Build history of the part. All positions in model axes, mm. A direction names the side the tool comes from. Give positions to 0.01 mm unless a question says otherwise; leave off trailing zeros. Order: outer loops, then holes, each group sorted by start corner. A loop starts at its lowest first (then second) coordinate and runs counter-clockwise, first axis right, second up. Notation, with made-up numbers: M 2.5,8.25 L 52.5,8.25 A6 ccw 52.5,13.25 Z; hole C 1.5,76 d8. An arc over 180 degrees is marked long. One line per item, written item: value. Start each with the question number.
from build123d import *

# Parameters (mm, degrees)
SKETCH1_W           = 92.3
SKETCH1_H           = 30.5
SKETCH1_W_2         = 84.3
SKETCH1_H_2         = 26.5
BOSS_EXTRUDE1_DEPTH = 3
SKETCH2_W           = 3
SKETCH2_H           = 3
BOSS_EXTRUDE2_DEPTH = 5


with BuildPart() as part:
    # Sketch1 → Boss-Extrude1 (new body)
    # profile 1 of 2: a face of its own
    with BuildSketch(Plane.XY):
        with Locations((0, 0.6)):
            Rectangle(SKETCH1_W, SKETCH1_H)
        with Locations((0, 0.6)):
            Rectangle(SKETCH1_W_2, SKETCH1_H_2, mode=Mode.SUBTRACT)
    # profile 2 of 2: a face of its own
    with BuildSketch(Plane.XY):
        with Locations((0, 0.6)):
            Rectangle(SKETCH1_W_2, SKETCH1_H_2)
    extrude(amount=BOSS_EXTRUDE1_DEPTH)

    # Sketch2 → Boss-Extrude2 (add)
    with BuildSketch(Plane.XY.offset(3)):
        with Locations((-40.65, 12.35)):
            Rectangle(SKETCH2_W, SKETCH2_H)
        with Locations((40.65, 12.35)):
            Rectangle(SKETCH2_W, SKETCH2_H)
        with Locations((40.65, -11.15)):
            Rectangle(SKETCH2_W, SKETCH2_H)
        with Locations((-40.65, -11.15)):
            Rectangle(SKETCH2_W, SKETCH2_H)
    extrude(amount=BOSS_EXTRUDE2_DEPTH)


solid = part.part
1) Drop flat-ended pins along their axis: P1, Ø1.5, axis at y = 12, z = 6, coming from the +X side; P2, Ø3.5, axis at x = -41.5, z = 5, coming from the +Y side; P3, Ø3.5, axis at x = -41, z = 6, coming from the -Y side. Give the stop position or say it passes through.
2) Slice it at A-A (z = 4.5). List the corners of the cut face in (x, y).
3) Pull direction Y, two halves, no side cores. Call faces 1 (the flat face through (41, 10.85, 5)), 2 (the flat face through (-1, -14.65, 1)), 3 (the flat face through (41, 13.85, 5)), 4 (the flat face through (46.15, 0, 1)): pulls with the +Y half, pulls with the -Y half, needs draft (parallel to the pull), parting line crosses it, or undercut.
4) Tool access for faces 5 (the flat face through (42.15, -11, 5)), 6 (the flat face through (-41, 13.85, 5)), 7 (the flat face through (-41, -12.65, 5)), 8 (the flat face through (39.15, -11, 5)): list every direction of +Z, -Z, +X, -X, +Y, -Y with a clear straight run to the whole face (end or side of a thin tool).
5) Slice it at B-B (y = 13). List the corners of the cut face in (x, z).
6) Slice it at C-C (x = 27.5). List the corners of the cut face in (y, z).
7) Drill centre lines: line 1 (X direction, y = 11, z = 4); line 2 (Z direction, x = -9.5, y = 6). Where is each one in solid material? Low to high.
8) Slice it at D-D (y = 2). List the corners of the cut face in (x, z), plus the area to 3 significant figures.
Results list:
1. P1: stops at x = 42.15
1. P2: stops at y = 13.85
1. P3: stops at y = -12.65
2. outline: M -42.15,-12.65 L -39.15,-12.65 L -39.15,-9.65 L -42.15,-9.65 Z; M -42.15,10.85 L -39.15,10.85 L -39.15,13.85 L -42.15,13.85 Z; M 39.15,-12.65 L 42.15,-12.65 L 42.15,-9.65 L 39.15,-9.65 Z; M 39.15,10.85 L 42.15,10.85 L 42.15,13.85 L 39.15,13.85 Z
3. face 1: undercut
3. face 2: pulls with the -Y half
3. face 3: pulls with the +Y half
3. face 4: needs draft
4. face 5: +Z, +X, +Y, -Y
4. face 6: +Z, +X, -X, +Y
4. face 7: +Z, +X, -X, -Y
4. face 8: +Z, +Y, -Y
5. outline: M -46.15,0 L 46.15,0 L 46.15,3 L 42.15,3 L 42.15,8 L 39.15,8 L 39.15,3 L -39.15,3 L -39.15,8 L -42.15,8 L -42.15,3 L -46.15,3 Z
6. outline: M -14.65,0 L 15.85,0 L 15.85,3 L -14.65,3 Z
7. line 1: x = -42.15 to -39.15, 39.15 to 42.15
7. line 2: z = 0 to 3
8. outline: M -46.15,0 L 46.15,0 L 46.15,3 L -46.15,3 Z
8. area: 277 mm²
